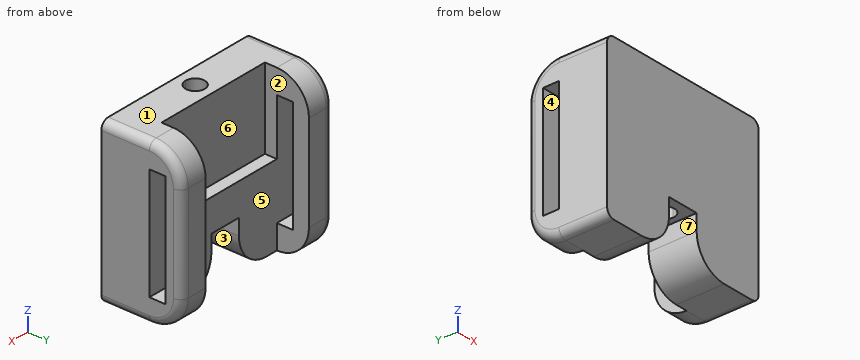
from build123d import *

# Parameters (mm, degrees)
SKETCH1_W           = 11
SKETCH1_H           = 10
BOSS_EXTRUDE1_DEPTH = 3
CUT_EXTRUDE4_DEPTH  = 12
CUT_EXTRUDE5_DEPTH  = 0.75
SKETCH6_W           = 1.75
SKETCH6_H           = 1.5
BOSS_EXTRUDE2_DEPTH = 1
SKETCH7_W           = 1.75
SKETCH7_H           = 10
BOSS_EXTRUDE3_DEPTH = 1
CUT_EXTRUDE6_DEPTH  = 12
FILLET4_R           = 2
FILLET5_R           = 2
FILLET6_R           = 0.5
FILLET7_R           = 0.5


with BuildPart() as part:
    # Sketch1 → Boss-Extrude1 (new body)
    with BuildSketch(Plane(origin=(0, 0, 0), x_dir=(1, 0, 0), z_dir=(0, 1, 0))):
        with Locations((-109.833038928, -31.060593966)):
            Rectangle(SKETCH1_W, SKETCH1_H)
    extrude(amount=BOSS_EXTRUDE1_DEPTH)

    # Sketch2 → Cut-Extrude4 (cut)
    with BuildSketch(Plane(origin=(0, 3, 0), x_dir=(1, 0, 0), z_dir=(0, 1, 0))):
        Polygon((-108.833038928, -26.060593966), (-110.833038928, -26.060593966), (-110.833038928, -29.060593966), (-109.833038928, -29.060593966), (-108.833038928, -29.060593966), align=None)
    extrude(amount=-CUT_EXTRUDE4_DEPTH, mode=Mode.SUBTRACT)

    # Sketch5 → Cut-Extrude5 (cut)
    with BuildSketch(Plane(origin=(0, 3, 0), x_dir=(1, 0, 0), z_dir=(0, 1, 0))):
        Polygon((-109.833038928, -36.060593966), (-113.583038928, -36.060593966), (-113.583038928, -31.060593966), (-106.083038928, -31.060593966), (-106.083038928, -36.060593966), align=None)
    extrude(amount=-CUT_EXTRUDE5_DEPTH, mode=Mode.SUBTRACT)

    # Sketch6 → Boss-Extrude2 (add)
    with BuildSketch(Plane(origin=(0, 3, 0), x_dir=(1, 0, 0), z_dir=(0, 1, 0))):
        with Locations((-114.458038928, -35.310593966)):
            Rectangle(SKETCH6_W, SKETCH6_H)
        with Locations((-114.458038928, -26.810593966)):
            Rectangle(SKETCH6_W, SKETCH6_H)
        with Locations((-105.208038928, -26.810593966)):
            Rectangle(SKETCH6_W, SKETCH6_H)
        with Locations((-105.208038928, -35.310593966)):
            Rectangle(SKETCH6_W, SKETCH6_H)
    extrude(amount=BOSS_EXTRUDE2_DEPTH)

    # Sketch7 → Boss-Extrude3 (add)
    with BuildSketch(Plane(origin=(0, 4, 0), x_dir=(1, 0, 0), z_dir=(0, 1, 0))):
        with Locations((-114.458038928, -31.060593966)):
            Rectangle(SKETCH7_W, SKETCH7_H)
        with Locations((-105.208038928, -31.060593966)):
            Rectangle(SKETCH7_W, SKETCH7_H)
    extrude(amount=BOSS_EXTRUDE3_DEPTH)

    # Sketch8 → Cut-Extrude6 (cut)
    with BuildSketch(Plane.XY.offset(36.060593966)):
        with BuildLine():
            ThreePointArc((-109.233038928, 1.125), (-109.40877486, 1.549264069), (-109.833038928, 1.725))
            Line((-109.833038928, 1.725), (-109.833038928, 0.525))
            ThreePointArc((-109.833038928, 0.525), (-109.40877486, 0.700735931), (-109.233038928, 1.125))
        make_face()
        with BuildLine():
            Line((-109.833038928, 0.525), (-109.833038928, 1.725))
            ThreePointArc((-109.833038928, 1.725), (-110.433038928, 1.125), (-109.833038928, 0.525))
        make_face()
    extrude(amount=-CUT_EXTRUDE6_DEPTH, mode=Mode.SUBTRACT)

    # Fillet4
    fillet4_edges = [part.edges().sort_by_distance(p)[0] for p in [
        (-110.833038928, 1.5, 26.060593966),
        (-108.833038928, 1.5, 26.060593966),
    ]]
    fillet(fillet4_edges, radius=FILLET4_R)

    # Fillet5
    fillet5_edges = [part.edges().sort_by_distance(p)[0] for p in [
        (-105.208038928, 5, 26.060593966),
        (-114.458038928, 5, 26.060593966),
        (-105.208038928, 5, 36.060593966),
        (-114.458038928, 5, 36.060593966),
    ]]
    fillet(fillet5_edges, radius=FILLET5_R)

    # Fillet6
    fillet6_edges = [part.edges().sort_by_distance(p)[0] for p in [
        (-104.333038928, 5, 31.060593966),
        (-104.333038928, 1.5, 26.060593966),
        (-104.333038928, 1.5, 36.060593966),
        (-104.333038928, 4.414213562, 35.474807528),
        (-104.333038928, 4.414213562, 26.646380403),
    ]]
    fillet(fillet6_edges, radius=FILLET6_R)

    # Fillet7
    fillet7_edges = [part.edges().sort_by_distance(p)[0] for p in [
        (-115.333038928, 5, 31.060593966),
        (-115.333038928, 1.5, 36.060593966),
        (-115.333038928, 1.5, 26.060593966),
        (-115.333038928, 4.414213562, 35.474807528),
        (-115.333038928, 4.414213562, 26.646380403),
    ]]
    fillet(fillet7_edges, radius=FILLET7_R)


solid = part.part
Check sheet for the modelled part. Datum: model origin and axes. Units: mm. Face numbers are marked on the shaded views. A direction names the side the tool comes from. Round coordinates to 2 decimals unless told otherwise and drop trailing zeros. Order: outer loops, then holes, each group sorted by start corner. A loop starts at its lowest first (then second) coordinate and runs counter-clockwise, first axis right, second up.
Q1. Set-up check for the marked faces 1, 2, 3 and 4: record each of +Z, -Z, +X, -X, +Y, -Y from which the full face is reachable in a straight line by a thin tool's end or side.
Filled sheet:
face 1: +Z, +X, -X, +Y, -Y
face 2: +Z, +Y
face 3: -Z, +Y, -Y
face 4: +X, -X
Q2. Cross-section at A-A, the plane z = 33. Enter the section's corners in (x, y) (3 decimals), plus the area to 3 significant figures.
Filled sheet:
outline: (-115.333, 0) - (-104.333, 0) - (-104.333, 3) - (-106.083, 3) - (-106.083, 2.25) - (-113.583, 2.25) - (-113.583, 3) - (-115.333, 3) - close; (-115.333, 4) - (-113.583, 4) - (-113.583, 5) - (-114.833, 5) arc R0.5 ccw to (-115.333, 4.5) - close; (-106.083, 4) - (-104.333, 4) - (-104.333, 4.5) arc R0.5 ccw to (-104.833, 5) - (-106.083, 5) - close; hole circle Ø1.2 at (-109.833, 1.125)
area: 29.6 mm2
Q3. Cross-section at D-D, the plane z = 28.5. Enter the section's corners in (x, y).
Filled sheet:
outline: (-115.33, 0) - (-110.83, 0) - (-110.83, 3) - (-115.33, 3) - close; (-115.33, 4) - (-113.58, 4) - (-113.58, 5) - (-114.83, 5) arc R0.5 ccw to (-115.33, 4.5) - close; (-108.83, 0) - (-104.33, 0) - (-104.33, 3) - (-108.83, 3) - close; (-106.08, 4) - (-104.33, 4) - (-104.33, 4.5) arc R0.5 ccw to (-104.83, 5) - (-106.08, 5) - close
Q4. Draft check along Y on the marked faces 5, 6 and 7. Enter one of: pulls with the +Y half, pulls with the -Y half, needs draft (parallel to the pull), parting line crosses it, or undercut.
Filled sheet:
face 5: undercut
face 6: pulls with the +Y half
face 7: needs draft
Q5. Cross-section at B-B, the plane x = -113.75. Enter the section's corners in (y, z), plus the area to 3 significant figures.
Filled sheet:
outline: (0, 26.06) - (3, 26.06) arc R2 ccw to (5, 28.06) - (5, 34.06) arc R2 ccw to (3, 36.06) - (0, 36.06) - close; hole (3, 27.56) - (4, 27.56) - (4, 34.56) - (3, 34.56) - close
area: 41.3 mm2
Q6. Cross-section at C-C, the plane y = 0.7. Enter the section's corners in (x, z).
Filled sheet:
outline: (-115.33, 26.56) arc R0.5 ccw to (-114.83, 26.06) - (-112.83, 26.06) arc R2 ccw to (-110.83, 28.06) - (-110.83, 29.06) - (-110.26, 29.06) - (-110.26, 36.06) - (-114.83, 36.06) arc R0.5 ccw to (-115.33, 35.56) - close; (-109.41, 29.06) - (-108.83, 29.06) - (-108.83, 28.06) arc R2 ccw to (-106.83, 26.06) - (-104.83, 26.06) arc R0.5 ccw to (-104.33, 26.56) - (-104.33, 35.56) arc R0.5 ccw to (-104.83, 36.06) - (-109.41, 36.06) - close
Q7. Depth check by flat-ended pin: P1, Ø0.8, axis at x = -105.5, y = 3.5, coming from the +Z side; P2, Ø3, axis at x = -110, z = 34.5, coming from the +Y side; P3, Ø0.8, axis at x = -114, y = 3.5, coming from the -Z side. Enter the tip coordinate at first touch or a pass-through.
Filled sheet:
P1: stops at z = 36.06
P2: stops at y = 2.25
P3: stops at z = 26.06
Q8. Scan lines: L1, parallel to Y at x = -106, z = 32; L2, parallel to X at y = 1.8, z = 28.25; L3, parallel to X at y = 4.05, z = 33. Record each from-to range of solid material in increasing order.
Filled sheet:
L1: y = 0 to 3, 4 to 5
L2: x = -115.33 to -110.83, -108.83 to -104.33
L3: x = -115.33 to -113.58, -106.08 to -104.33
